Verification items for the finished model (mm, model axes). Give positions to 0.01 mm unless a question says otherwise; leave off trailing zeros. Write each loop counter-clockwise with the first axis right and the second up, starting at its lowest first coordinate (ties: lowest second). Pieces come first, ordered by that corner, then holes. Notation, with made-up numbers: (-10, 31.5) - (48, 31.5) arc R7 ccw to (48, 41.5) - close; hole circle Ø3 at (5.25, -27). An arc over 180 degrees is marked (long way). Answer as a JSON object with one key per item and string values. Group by question number.
Item 1: Sectioned sample at C-C, the plane z = 1.75. Count the separate pieces of the cut face and the enclosed holes in it, and give its area (3 significant figures).
Item 2: Go/stop test with flat-tipped pins: pin 1 (5 mm diameter, centred on y = 4.5, z = 4, fed in from -X); pin 2 (5 mm diameter, centred on y = 0.5, z = 5.5, fed in from +X); pin 3 (6 mm diameter, centred on x = 60, y = 22, fed in from -Z); pin 4 (3 mm diameter, centred on x = -44.5, y = -27, fed in from +Z) (3 decimals). Record where each tip stops, or that it passes through.
Item 3: Sectioned sample at A-A, the plane y = 6. Record the boundary of the cut face in (x, z) (3 decimals).
Item 4: Sectioned sample at B-B, the plane x = -128. Record the boundary of the cut face in (y, z) (1 decimal).
Item 5: Sectioned sample at D-D, the plane x = 156.5. Record the boundary of the cut face in (y, z) (1 decimal).
Item 6: Scan lines: line 1 along Y through (x, z) = (-69.5, 9.25); line 2 along X through (y, z) = (-1.5, 6.25); line 3 along X through (y, z) = (-8.5, 3.75). Record each from-to range of solid material in increasing order. Write a range as [from, to].
Autodesk Inventor part; units mm, degrees
ref_plane "YZ Plane" through (0, 0, 0) normal (1, 0, 0) x (0, 1, 0)
ref_plane "XZ Plane" through (0, 0, 0) normal (0, 1, 0) x (-1, 0, 0)
ref_plane "XY Plane" through (0, 0, 0) normal (0, 0, 1) x (1, 0, 0)
sketch "Sketch1" plane through (0, 0, 0) normal (0, 0, 1) x (1, 0, 0)
  line L0 (-56.2006, 27.4418) -> (-175.6588, 27.4418)
  line L1 (-56.2006, -15.6625) -> (-175.6588, -15.6625)
  line L2 (-48.2006, -7.6625) -> (-48.2006, 19.4418)
  line L3 (-183.6588, -7.6625) -> (-183.6588, 19.4418)
  line L4 (-286.5288, -19.4915) -> (-213.2441, -19.4915)
  line L5 (-286.5288, 31.2885) -> (-213.2441, 31.2885)
  line L6 (-205.2441, 23.2885) -> (-205.2441, -11.4915)
  line L7 (51.9852, 27.4415) -> (171.5472, 27.4415)
  line L8 (51.9852, -15.6445) -> (171.5472, -15.6445)
  line L9 (43.9852, 19.4415) -> (43.9852, -7.6445)
  line L10 (179.5472, 19.4415) -> (179.5472, -7.6445)
  arc A0 (-205.2441, 23.2885) -> (-213.2441, 31.2885) centre (-213.2441, 23.2885) ccw
  arc A1 (-175.6588, 27.4418) -> (-183.6588, 19.4418) centre (-175.6588, 19.4418) ccw
  arc A2 (-183.6588, -7.6625) -> (-175.6588, -15.6625) centre (-175.6588, -7.6625) ccw
  arc A3 (-56.2006, -15.6625) -> (-48.2006, -7.6625) centre (-56.2006, -7.6625) ccw
  arc A4 (-48.2006, 19.4418) -> (-56.2006, 27.4418) centre (-56.2006, 19.4418) ccw
  arc A5 (-213.2441, -19.4915) -> (-205.2441, -11.4915) centre (-213.2441, -11.4915) ccw
  arc A6 (51.9852, 27.4415) -> (43.9852, 19.4415) centre (51.9852, 19.4415) ccw
  arc A7 (43.9852, -7.6445) -> (51.9852, -15.6445) centre (51.9852, -7.6445) ccw
  arc A8 (171.5472, -15.6445) -> (179.5472, -7.6445) centre (171.5472, -7.6445) ccw
  arc A9 (179.5472, 19.4415) -> (171.5472, 27.4415) centre (171.5472, 19.4415) ccw
  line L11 (-286.5288, 50.3385) -> (282.4312, 50.3385)
  line L12 (-286.5288, -38.5415) -> (282.4312, -38.5415)
  line L13 (-286.5288, 31.2885) -> (-286.5288, 50.3385)
  line L14 (-286.5288, -19.4915) -> (-286.5288, -38.5415)
  line L15 (179.5472, 5.8985) -> (201.1322, 5.9085)
  line L16 (282.4312, 31.2885) -> (209.1322, 31.2885)
  line L17 (201.1322, 23.2885) -> (201.1322, -11.4915)
  line L18 (209.1322, -19.4915) -> (282.4312, -19.4915)
  arc A10 (201.1322, -11.4915) -> (209.1322, -19.4915) centre (209.1322, -11.4915) ccw
  arc A11 (209.1322, 31.2885) -> (201.1322, 23.2885) centre (209.1322, 23.2885) ccw
  line L19 (282.4312, 50.3385) -> (282.4312, 31.2885)
  line L20 (282.4312, -19.4915) -> (282.4312, -38.5415)
  point P0 (0, 0)
  point P1 (0, 0)
  point P2 (-209.4751, 31.2885)
  point P3 (-205.2441, 26.6389)
  point P4 (-209.4751, -19.4915)
  point P5 (-179.9924, 27.4418)
  point P6 (-183.6588, 23.2495)
  point P7 (-183.6588, -11.4325)
  point P8 (-179.4288, -15.6625)
  point P9 (-48.2006, 23.2495)
  point P10 (-52.4306, 27.4418)
  point P11 (-52.9924, -15.6625)
  point P12 (-48.2006, -11.4325)
  point P13 (-205.2441, -15.2625)
  point P14 (48.2152, 27.4415)
  point P15 (43.9852, 23.2115)
  point P16 (48.2152, -15.6445)
  point P17 (179.5472, 23.2115)
  point P18 (175.3172, 27.4415)
  point P19 (175.3172, -15.6445)
  point P20 (179.5472, -11.4145)
  point P21 (43.9852, -11.4145)
  dimension "d0" = 135.4582
  dimension "d1" = 43.1043
  dimension "d4" = 21.5853
  dimension "d5" = 92.1858
  dimension "d8" = 8
  dimension "d9" = 8
  dimension "d10" = 8
  dimension "d50" = 50.7799
  dimension "d62" = 88.8799
  dimension "d63" = 19.05
  dimension "d64" = 50.7799
ref_plane "Work Plane7" through (0, 0, 9.525) normal (0, 0, 1) x (1, 0, 0)
extrude "Extrusion6" add sketch "Sketch1" along normal blind 9.525
sketch "Sketch7" plane through (0, 0, 9.525) normal (0, 0, 1) x (1, 0, 0)
  line L0 (-286.5288, 50.3385) -> (-286.5288, 31.2885)
  line L1 (282.4312, 31.2885) -> (282.4312, 50.3385)
  line L2 (-286.5288, 45.576) -> (282.4312, 45.576)
  line L3 (282.4312, 45.576) -> (282.4312, 36.051)
  line L4 (282.4312, 36.051) -> (-286.5288, 36.051)
  line L5 (-286.5288, 36.051) -> (-286.5288, 45.576)
  line L6 (282.4312, 50.3385) -> (-286.5288, 50.3385)
  line L7 (282.4312, -38.5415) -> (282.4312, -19.4915)
  line L8 (-286.5288, -24.254) -> (282.4312, -24.254)
  line L9 (282.4312, -24.254) -> (282.4312, -33.779)
  line L10 (282.4312, -33.779) -> (-286.5288, -33.779)
  line L11 (-286.5288, -33.779) -> (-286.5288, -24.254)
  line L12 (-286.5288, -38.5415) -> (282.4312, -38.5415)
  point P0 (0, 0)
  dimension "d98" = 9.525
  dimension "d99" = 4.7625
  dimension "d100" = 4.7625
  dimension "d101" = 9.525
emboss "Emboss7" sketch "Sketch7" operation cut depth 3 direction (0, 0, -1) contours L2 L1 L4 L0 | L10 L11 L8 L7
properties part number "top" material "Aluminum 6061"
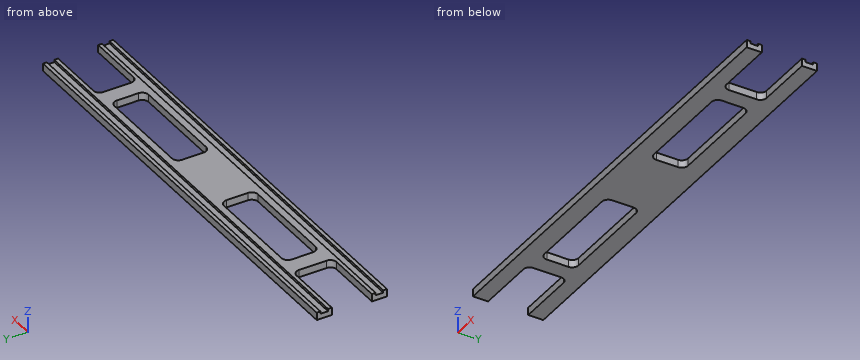
Geometry check:
{
 "1": {"separate pieces": "1", "enclosed holes": "2", "area": "30,800 mm^2"},
 "2": {"pin 1": "x = -205.24", "pin 2": "x = 201.13", "pin 3": "through", "pin 4": "z = 6.525"},
 "3": {"outline": "(-205.244, 0) - (-183.659, 0) - (-183.659, 9.525) - (-205.244, 9.525) - close; (-48.201, 0) - (43.985, 0) - (43.985, 9.525) - (-48.201, 9.525) - close; (179.547, 0) - (201.132, 0) - (201.132, 9.525) - (179.547, 9.525) - close"},
 "4": {"outline": "(-38.5, 0) - (-15.7, 0) - (-15.7, 9.5) - (-24.3, 9.5) - (-24.3, 6.5) - (-33.8, 6.5) - (-33.8, 9.5) - (-38.5, 9.5) - close; (27.4, 0) - (50.3, 0) - (50.3, 9.5) - (45.6, 9.5) - (45.6, 6.5) - (36.1, 6.5) - (36.1, 9.5) - (27.4, 9.5) - close"},
 "5": {"outline": "(-38.5, 0) - (-15.6, 0) - (-15.6, 9.5) - (-24.3, 9.5) - (-24.3, 6.5) - (-33.8, 6.5) - (-33.8, 9.5) - (-38.5, 9.5) - close; (27.4, 0) - (50.3, 0) - (50.3, 9.5) - (45.6, 9.5) - (45.6, 6.5) - (36.1, 6.5) - (36.1, 9.5) - (27.4, 9.5) - close"},
 "6": {"line 1": "[-38.54, -33.78], [-24.25, -15.66], [27.44, 36.05], [45.58, 50.34]", "line 2": "[-205.24, -183.66], [-48.2, 43.99], [179.55, 201.13]", "line 3": "[-205.24, -183.61], [-48.24, 44.03], [179.5, 201.13]"}
}
